```python
from build123d import *

# Parameters (mm, degrees)
SKETCH1_W           = 1094.236516538
SKETCH1_H           = 400
BOSS_EXTRUDE1_DEPTH = 18
CAVITY1_START       = -15
CAVITY1_OUTLINE_W   = 18
CAVITY1_OUTLINE_H   = 18
CAVITY1_DEPTH       = 30
CAVITY1_START_2     = 813.236516538
CAVITY1_2_OUTLINE_W = 18
CAVITY1_2_OUTLINE_H = 18
CAVITY1_2_DEPTH     = 30
CAVITY1_START_3     = 389.118258269
CAVITY1_3_OUTLINE_W = 18
CAVITY1_3_OUTLINE_H = 18
CAVITY1_3_DEPTH     = 50
CAVITY1_START_4     = -35
CAVITY1_4_OUTLINE_W = 18
CAVITY1_4_OUTLINE_H = 18
CAVITY1_4_DEPTH     = 20
CAVITY1_START_5     = 15
CAVITY1_5_OUTLINE_W = 18
CAVITY1_5_OUTLINE_H = 18
CAVITY1_5_DEPTH     = 20
CAVITY1_START_6     = 793.236516538
CAVITY1_6_OUTLINE_W = 18
CAVITY1_6_OUTLINE_H = 18
CAVITY1_6_DEPTH     = 20
CAVITY1_START_7     = 843.236516538
CAVITY1_7_OUTLINE_W = 18
CAVITY1_7_OUTLINE_H = 18
CAVITY1_7_DEPTH     = 20
SKETCH2_W           = 18
SKETCH2_H           = 50
CUT_EXTRUDE1_DEPTH  = 987.255362837
SKETCH3_W           = 798.236516538
SKETCH3_H           = 209.4
CUT_EXTRUDE2_DEPTH  = 18


# Read off the part's stored shape, not the designer's step: Cavity1
with BuildPart() as part:
    # Sketch1 → Boss-Extrude1 (new body)
    with BuildSketch(Plane.XY):
        with Locations((414.118258269, 20)):
            Rectangle(SKETCH1_W, SKETCH1_H)
    extrude(amount=BOSS_EXTRUDE1_DEPTH)

    # Cavity1 outline → Cavity1 (cut)
    with BuildSketch(Plane.YZ.offset(CAVITY1_START)):
        with Locations((-9, 9)):
            Rectangle(CAVITY1_OUTLINE_W, CAVITY1_OUTLINE_H)
        with Locations((-171, 9)):
            Rectangle(CAVITY1_OUTLINE_W, CAVITY1_OUTLINE_H)
    extrude(amount=CAVITY1_DEPTH, mode=Mode.SUBTRACT)

    # Cavity1 2 outline → Cavity1 2 (cut)
    with BuildSketch(Plane.YZ.offset(CAVITY1_START_2)):
        with Locations((-9, 9)):
            Rectangle(CAVITY1_2_OUTLINE_W, CAVITY1_2_OUTLINE_H)
        with Locations((-171, 9)):
            Rectangle(CAVITY1_2_OUTLINE_W, CAVITY1_2_OUTLINE_H)
    extrude(amount=CAVITY1_2_DEPTH, mode=Mode.SUBTRACT)

    # Cavity1 3 outline → Cavity1 3 (cut)
    with BuildSketch(Plane.YZ.offset(CAVITY1_START_3)):
        with Locations((-171, 9)):
            Rectangle(CAVITY1_3_OUTLINE_W, CAVITY1_3_OUTLINE_H)
    extrude(amount=CAVITY1_3_DEPTH, mode=Mode.SUBTRACT)

    # Cavity1 4 outline → Cavity1 4 (cut)
    with BuildSketch(Plane.YZ.offset(CAVITY1_START_4)):
        with Locations((-9, 9)):
            Rectangle(CAVITY1_4_OUTLINE_W, CAVITY1_4_OUTLINE_H)
    extrude(amount=CAVITY1_4_DEPTH, mode=Mode.SUBTRACT)

    # Cavity1 5 outline → Cavity1 5 (cut)
    with BuildSketch(Plane.YZ.offset(CAVITY1_START_5)):
        with Locations((-171, 9)):
            Rectangle(CAVITY1_5_OUTLINE_W, CAVITY1_5_OUTLINE_H)
    extrude(amount=CAVITY1_5_DEPTH, mode=Mode.SUBTRACT)

    # Cavity1 6 outline → Cavity1 6 (cut)
    with BuildSketch(Plane.YZ.offset(CAVITY1_START_6)):
        with Locations((-171, 9)):
            Rectangle(CAVITY1_6_OUTLINE_W, CAVITY1_6_OUTLINE_H)
    extrude(amount=CAVITY1_6_DEPTH, mode=Mode.SUBTRACT)

    # Cavity1 7 outline → Cavity1 7 (cut)
    with BuildSketch(Plane.YZ.offset(CAVITY1_START_7)):
        with Locations((-9, 9)):
            Rectangle(CAVITY1_7_OUTLINE_W, CAVITY1_7_OUTLINE_H)
    extrude(amount=CAVITY1_7_DEPTH, mode=Mode.SUBTRACT)

    # Sketch2 → Cut-Extrude1 (cut, through all)
    with BuildSketch(Plane.XY.offset(18)):
        with Locations((952.236516538, 145)):
            Rectangle(SKETCH2_W, SKETCH2_H)
        with Locations((952.236516538, -105)):
            Rectangle(SKETCH2_W, SKETCH2_H)
        with Locations((-124, -105)):
            Rectangle(SKETCH2_W, SKETCH2_H)
        with Locations((-124, 145)):
            Rectangle(SKETCH2_W, SKETCH2_H)
    extrude(amount=-CUT_EXTRUDE1_DEPTH, mode=Mode.SUBTRACT)

    # Sketch3 → Cut-Extrude2 (cut)
    with BuildSketch(Plane.XY.offset(18)):
        with Locations((414.118258269, 115.3)):
            Rectangle(SKETCH3_W, SKETCH3_H)
    extrude(amount=-CUT_EXTRUDE2_DEPTH, mode=Mode.SUBTRACT)


solid = part.part
```
Input: part model. Units: mm. Frame: model coordinates. A direction names the side the tool comes from. Coordinates: 2 decimals unless noted, no trailing zeros. Loops run counter-clockwise (first coordinate to the right, second up) from the corner with the lowest first, then second, coordinate; pieces in that order, holes last. Notation, with made-up numbers: M 63.25,-23 L 73.25,-23 A24 ccw 73.25,12 Z; hole C 65,36.25 d5. An arc over 180 degrees is marked long. Use a Markdown table: item, result. Add a question column.
1) Line query: L1, parallel to X at y = 189.5, z = 12; L2, parallel to X at y = 147.5, z = 7.75; L3, parallel to Y at x = 83, z = 9.5. Output: solid intervals per line, ascending. Write a range as from..to.
2) Draft query along Y for faces 5 (the flat face through (961.237, 19, 9)), 6 (the flat face through (838, 0, 9)), 7 (the flat face through (210, -180, 9)), 8 (the flat face through (-115, 145, 9)). Return one class per face: +Y half, -Y half, draft (parallel to the pull), parting line (faces both ways), or undercut.
3) Pin query (flat end, axial travel): P1, Ø5.5, axis at y = 147.5, z = 13.5, coming from the +X side; P2, Ø5, axis at x = 478, z = 14, coming from the +Y side; P3, Ø5.5, axis at y = 154, z = 12, coming from the -X side. Return the tip coordinate at first contact, or that it passes through.
4) Section C-C, the plane x = 426. Return the cut outline in (y, z), plus the area to 3 significant figures.
5) Section B-B, the plane y = 155. Return the cut outline in (x, z), plus the area to 3 significant figures.
6) Set-up query: faces 1 (the flat face through (414, -162, 9)), 2 (the flat face through (943.237, -105, 9)), 3 (the flat face through (863.237, -9, 9)), 4 (the flat face through (-115, -105, 9)). Return all of +Z, -Z, +X, -X, +Y, -Y with unobstructed straight access to the full face (end or side cutting, diameter ignored); none if empty.
7) Section A-A, the plane y = 82.5. Return the cut outline in (x, z).
8) Section D-D, the plane z = 14. Give the number of separate pieces and of enclosed holes in the cut face, plus the area to 3 significant figures.
Answer below:
| question | item | result |
|---|---|---|
| 1 | L1 | -133..15, 813.24..961.24 |
| 1 | L2 | -115..15, 813.24..943.24 |
| 1 | L3 | -180..10.6 |
| 2 | face 5 | draft |
| 2 | face 6 | undercut |
| 2 | face 7 | -Y half |
| 2 | face 8 | undercut |
| 3 | P1 | x = 943.24 |
| 3 | P2 | y = 10.6 |
| 3 | P3 | x = -115 |
| 4 | outline | M -162,0 L 10.6,0 L 10.6,18 L -162,18 Z |
| 4 | area | 3,110 mm2 |
| 5 | outline | M -115,0 L 15,0 L 15,18 L -115,18 Z; M 813.24,0 L 943.24,0 L 943.24,18 L 813.24,18 Z |
| 5 | area | 4,680 mm2 |
| 6 | face 1 | +Z, -Z, -Y |
| 6 | face 2 | +Z, -Z, +X |
| 6 | face 3 | +Z, -Z |
| 6 | face 4 | +Z, -Z, -X |
| 7 | outline | M -133,0 L 15,0 L 15,18 L -133,18 Z; M 813.24,0 L 961.24,0 L 961.24,18 L 813.24,18 Z |
| 8 | separate pieces | 1 |
| 8 | enclosed holes | 2 |
| 8 | area | 262,000 mm2 |
